```python
from build123d import *


with BuildPart() as f1:
    # F0 (on Top) → F1 (revolve)
    with BuildSketch(Plane.XY):
        with BuildLine():
            Line((-36.538901, 10), (-46.538901, 10))
            Line((-46.538901, 10), (-46.538901, 0))
            Line((-46.538901, 0), (123.461099, 0))
            Line((123.461099, 0), (123.461099, 10))
            Line((123.461099, 10), (113.461099, 10))
            add(Edge.make_bspline(
                [(78.461099, 30), (89.132972, 30), (102.789225, 10), (113.461099, 10)],
                knots=[0, 0, 0, 0, 40.311289, 40.311289, 40.311289, 40.311289], degree=3))
            Line((78.461099, 30), (-1.538901, 30))
            add(Edge.make_bspline(
                [(-1.538901, 30), (-12.210775, 30), (-25.867028, 10), (-36.538901, 10)],
                knots=[0, 0, 0, 0, 40.311289, 40.311289, 40.311289, 40.311289], degree=3))
        make_face()
    revolve(axis=Axis((15.960287, 0, 0), (1, 0, 0)))


solid = f1.part
```
Here's how the part is built. I have some questions about the finished solid (model axes, mm). A direction names the side the tool comes from. Coordinates: 2 decimals unless noted, no trailing zeros. Order: outer loops, then holes, each group sorted by start corner. A loop starts at its lowest first (then second) coordinate and runs counter-clockwise, first axis right, second up. Notation, with made-up numbers: (-7, 67.5) - (11, 67.5) arc R25 ccw to (11, 79.5) - close; hole circle Ø10 at (17.25, -38). An arc over 180 degrees is marked (long way). One line per question, with ' | ' between items. Start each with the question number.
1. If we section it at A-A (x = 26): Write out the boundary of the cut face in (y, z).
2. I'm going to push flat-ended pins straight in: pin 1 Ø10 at (x, z) = (5.5, 7.5) entering from +Y; pin 2 Ø12 at (x, y) = (104, -9) entering from +Z; pin 3 Ø8 at (x, z) = (46, 13) entering from -Y. Where does each tip first touch, or does it pass through?
3. Please list where these lines run through material, in increasing order: line 1 along X through (y, z) = (-6, -20); line 2 along X through (y, z) = (3, 26.5); line 3 along Z through (x, y) = (14, -2). Write a range as [from, to].
4. Which directions (+Z, -Z, +X, -X, +Y, -Y) give clear straight access to the entire face, cutting with the end or side of a thin tool? Please do faces 1 (the cylindrical face through (-41.61, -2.17, -9.76)), 2 (the cylindrical face through (37.9, -29.97, 1.32)), 3 (the cylindrical face through (118.39, -2.17, -9.76)).
Model answer:
1) outline: circle Ø60 at (0, 0)
2) pin 1: stops at y = 29.9 | pin 2: stops at z = 16.67 | pin 3: stops at y = -28.62
3) line 1: x = [-17.97, 94.89] | line 2: x = [-10.33, 87.25] | line 3: z = [-29.93, 29.93]
4) face 1: -X | face 2: +X, -X | face 3: +X
